```python
from build123d import *

# Parameters (mm, degrees)
BOSS_EXTRUDE1_DEPTH = 13.5
CUT_EXTRUDE1_DEPTH  = 19.454335534
SKETCH14_R          = 1.65
SKETCH14_R_2        = 1.483994527
BOSS_EXTRUDE3_DEPTH = 9.4
CUT_EXTRUDE7_DEPTH  = 43.344584395
FILLET2_R           = 2
CUT_EXTRUDE8_DEPTH  = 4
CUT_EXTRUDE9_DEPTH  = 5.4
CHAMFER2_SIZE       = 12
CHAMFER2_SIZE_2     = 6
CHAMFER3_SIZE       = 6
CHAMFER3_SIZE_2     = 12
SKETCH18_R          = 14.026707194
CUT_EXTRUDE10_DEPTH = 3
CUT_EXTRUDE11_DEPTH = 1


with BuildPart() as part:
    # Sketch1 → Boss-Extrude1 (new body)
    with BuildSketch(Plane.ZY):
        with BuildLine():
            Line((-9.5, 8.25), (-9.5, -8.25))
            Line((-9.5, -8.25), (0, -8.25))
            ThreePointArc((0, -8.25), (8.25, 0), (0, 8.25))
            Line((0, 8.25), (-9.5, 8.25))
        make_face()
    extrude(amount=BOSS_EXTRUDE1_DEPTH)

    # Sketch7 → Cut-Extrude1 (cut, through all)
    with BuildSketch(Plane.ZY.offset(13.5)):
        with BuildLine():
            Line((13.481907846, 13.481907846), (4.313351365, 4.313351365))
            ThreePointArc((4.313351365, 4.313351365), (-5.89214754, 1.578796175), (1.578796175, -5.89214754))
            Line((1.578796175, -5.89214754), (4.934720763, -18.416628609))
            Line((4.934720763, -18.416628609), (13.481907846, 13.481907846))
        make_face()
    extrude(amount=-CUT_EXTRUDE1_DEPTH, mode=Mode.SUBTRACT)

    # Sketch14 → Boss-Extrude3 (add)
    with BuildSketch(Plane(origin=(0, 0, -9.5), x_dir=(-1, 0, 0), z_dir=(0, 0, -1))):
        with BuildLine():
            Line((4.039848555, 24.201794753), (-19.358847021, 9.109670469))
            Line((-19.358847021, 9.109670469), (-19.131451731, 4.496469334))
            Line((-19.131451731, 4.496469334), (-15.022604709, 2.386798865))
            Line((-15.022604709, 2.386798865), (0, 12.07635684))
            Line((0, 12.07635684), (0, 8.25))
            Line((0, 8.25), (13.5, 8.25))
            Line((13.5, 8.25), (13.5, 12.07635684))
            Line((13.5, 12.07635684), (28.522604709, 2.386798865))
            Line((28.522604709, 2.386798865), (32.631451731, 4.496469334))
            Line((32.631451731, 4.496469334), (32.858847021, 9.109670469))
            Line((32.858847021, 9.109670469), (9.460151445, 24.201794753))
            ThreePointArc((9.460151445, 24.201794753), (6.75, 25), (4.039848555, 24.201794753))
        make_face()
        with Locations((6.75, 20)):
            Circle(SKETCH14_R, mode=Mode.SUBTRACT)
        with Locations((-15.25, 7)):
            Circle(SKETCH14_R_2, mode=Mode.SUBTRACT)
        with Locations(Location((28.75, 7, 0), (0, 0, 180))):
            Circle(SKETCH14_R_2, mode=Mode.SUBTRACT)
    extrude(amount=-BOSS_EXTRUDE3_DEPTH)

    # Sketch15 → Cut-Extrude7 (cut, through all)
    with BuildSketch(Plane.XY.offset(-0.1)):
        Polygon((0, 8.25), (-10.401710887, 8.25), (0, 10.084102275), align=None)
        Polygon((-13.5, 10.242254565), (-13.5, 12.07635684), (-3.098289113, 12.07635684), align=None)
    extrude(amount=-CUT_EXTRUDE7_DEPTH, mode=Mode.SUBTRACT)

    # Fillet2
    fillet2_edges = [part.edges().sort_by_distance(p)[0] for p in [
        (0, 10.084102275, -4.8),
        (-13.5, 10.242254565, -4.8),
    ]]
    fillet(fillet2_edges, radius=FILLET2_R)

    # Sketch16 → Cut-Extrude8 (cut)
    with BuildSketch(Plane(origin=(0, 0, -9.5), x_dir=(-1, 0, 0), z_dir=(0, 0, -1))):
        Polygon((6.75, 16.651368439), (9.65, 18.325684219), (9.65, 21.674315781), (6.75, 23.348631561), (3.85, 21.674315781), (3.85, 18.325684219), align=None)
    extrude(amount=-CUT_EXTRUDE8_DEPTH, mode=Mode.SUBTRACT)

    # Sketch17 → Cut-Extrude9 (cut)
    with BuildSketch(Plane.XY.offset(-0.1)):
        with BuildLine():
            Line((19.131451731, 4.496469334), (19.358847021, 9.109670469))
            Line((19.358847021, 9.109670469), (17.418121156, 10.361435802))
            ThreePointArc((17.418121156, 10.361435802), (11.888564198, 9.168121156), (13.081878844, 3.638564198))
            Line((13.081878844, 3.638564198), (15.022604709, 2.386798865))
            Line((15.022604709, 2.386798865), (19.131451731, 4.496469334))
        make_face()
        with BuildLine():
            Line((-32.631451731, 4.496469334), (-28.522604709, 2.386798865))
            Line((-28.522604709, 2.386798865), (-26.581878844, 3.638564198))
            ThreePointArc((-26.581878844, 3.638564198), (-25.388564198, 9.168121156), (-30.918121156, 10.361435802))
            Line((-30.918121156, 10.361435802), (-32.858847021, 9.109670469))
            Line((-32.858847021, 9.109670469), (-32.631451731, 4.496469334))
        make_face()
    extrude(amount=-CUT_EXTRUDE9_DEPTH, mode=Mode.SUBTRACT)

    # Chamfer2
    # the kernel refuses this chamfer: 12, 6 mm, written as the material it takes off along each edge
    with BuildSketch(Plane(origin=(-28.75, 7, -0.1), x_dir=(-0.8386519680093931, -0.5446676753342096, 0), z_dir=(-0.5446676753342096, 0.8386519680093931, 0))) as chamfer2_piece_1_section:
        Polygon((4 + CHAMFER2_SIZE, 0), (4, -CHAMFER2_SIZE_2), (4, 0), align=None)
    chamfer2_piece_1 = revolve(axis=Axis((-28.75, 7, -0.1), (0, 0, 1)), revolution_arc=359.64, mode=Mode.PRIVATE)
    chamfer2_piece_1 = split(chamfer2_piece_1, bisect_by=Plane(origin=(-24.520519127, 4.968138188, -1.544016366), z_dir=(-0.5420302889814643, 0.8403589505840171, 0)), keep=Keep.TOP, mode=Mode.PRIVATE)
    chamfer2_piece_1 = split(chamfer2_piece_1, bisect_by=Plane(origin=(-24.679235885, 5.214211241, -5.5), z_dir=(0, 0, 1)), keep=Keep.TOP, mode=Mode.PRIVATE)
    add(chamfer2_piece_1, mode=Mode.SUBTRACT)

    # Chamfer3
    # the kernel refuses this chamfer: 12, 6 mm, written as the material it takes off along each edge
    with BuildSketch(Plane(origin=(15.25, 7, -0.1), x_dir=(0.8420576391550663, -0.5393875530085916, 0), z_dir=(-0.5393875530085916, -0.8420576391550663, 0))) as chamfer3_piece_1_section:
        Polygon((4, -CHAMFER3_SIZE), (4 + CHAMFER3_SIZE_2, 0), (4, 0), align=None)
    chamfer3_piece_1 = revolve(axis=Axis((15.25, 7, -0.1), (0, 0, 1)), revolution_arc=359.64, mode=Mode.PRIVATE)
    chamfer3_piece_1 = split(chamfer3_piece_1, bisect_by=Plane(origin=(8.890128565, 11.795128101, -5.5), z_dir=(0, 0, 1)), keep=Keep.TOP, mode=Mode.PRIVATE)
    chamfer3_piece_1 = split(chamfer3_piece_1, bisect_by=Plane(origin=(0, 11.795128101, -1.99911645), z_dir=(1, 0, 0)), keep=Keep.TOP, mode=Mode.PRIVATE)
    add(chamfer3_piece_1, mode=Mode.SUBTRACT)

    # Sketch18 → Cut-Extrude10 (cut)
    with BuildSketch(Plane.XY.offset(-0.1)):
        with Locations((-6.75, 28.841468874)):
            Circle(SKETCH18_R)
    extrude(amount=-CUT_EXTRUDE10_DEPTH, mode=Mode.SUBTRACT)

    # Sketch19 → Cut-Extrude11 (cut)
    with BuildSketch(Plane.XY.offset(-5.5)):
        Polygon((-31.564052505, 5.184940267), (-28.585138414, 3.655429177), (-25.77108591, 5.47048891), (-25.935947495, 8.815059733), (-28.914861586, 10.344570823), (-31.72891409, 8.52951109), align=None)
        Polygon((18.064052505, 5.184940267), (18.22891409, 8.52951109), (15.414861586, 10.344570823), (12.435947495, 8.815059733), (12.27108591, 5.47048891), (15.085138414, 3.655429177), align=None)
    extrude(amount=-CUT_EXTRUDE11_DEPTH, mode=Mode.SUBTRACT)


solid = part.part
```
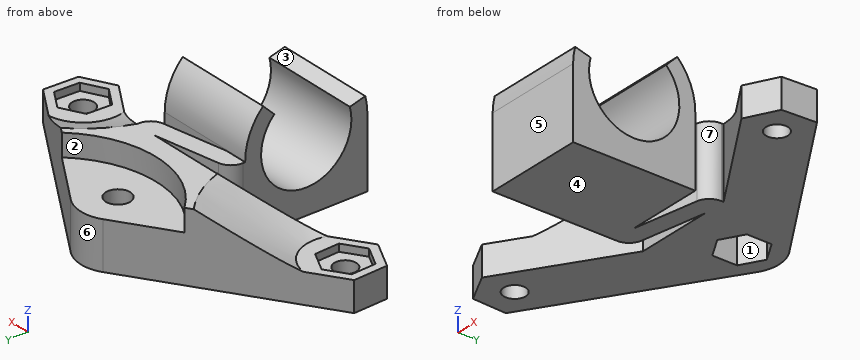
Check sheet for the modelled part. Datum: model origin and axes. Units: mm. Face numbers are marked on the shaded views. A direction names the side the tool comes from. Round coordinates to 2 decimals unless told otherwise and drop trailing zeros. Loops run counter-clockwise (first coordinate to the right, second up) from the corner with the lowest first, then second, coordinate; pieces in that order, holes last. Notation, with made-up numbers: (12, 24.5) -> (50, 24.5) arc R29 ccw to (50, 63.5) -> close; hole circle Ø11 at (-39, 72). An arc over 180 degrees is marked (long way). Write item = value, one per line. Start each with the question number.
1) Sectioned sample at B-B, the plane y = 20. Record the cut outline in (x, z).
2) Thickness scan on probe 1 along X at (y, z) = (8, -7); probe 2 along X at (y, z) = (-7, -1.5); probe 3 along Z at (x, y) = (-3, 0). Record the ranges inside material, lowest first.
3) Release check for a two-part mould opening along Y. For the marked faces 4, 5, 6 and 7 record: released by +Y, released by -Y, zero draft, split by the parting line, or undercut.
4) Gauge pin test, flat ends, axial feed: pin 1 Ø5 at (x, y) = (-7, 18) entering from +Z; pin 2 Ø1 at (x, y) = (-23, 10.5) entering from +Z; pin 3 Ø9 at (x, y) = (-10, 14) entering from +Z. Record the tip position at first contact, or that the pin passes through.
5) Set-up check for the marked faces 1, 2 and 3: record each of +Z, -Z, +X, -X, +Y, -Y from which the full face is reachable in a straight line by a thin tool's end or side.
6) Sectioned sample at D-D, the plane y = 0. Record the cut outline in (x, z).
7) Sectioned sample at C-C, the plane y = 7. State how many separate pieces and enclosed holes the cut face has, plus the area to 3 significant figures.
8) Sectioned sample at A-A, the plane z = -4. Record the cut outline in (x, y), plus the area to 3 significant figures.
Results are:
q1.outline = (-15.97, -9.5) -> (-9.65, -9.5) -> (-9.65, -5.5) -> (-8.4, -5.5) -> (-8.4, -3.1) -> (-15.97, -3.1) -> close; (-5.1, -5.5) -> (-3.85, -5.5) -> (-3.85, -9.5) -> (2.47, -9.5) -> (2.47, -3.1) -> (-5.1, -3.1) -> close
q2.probe_1 = -32.8 to -29.85, -27.65 to -19.82, -13.5 to 0, 6.32 to 14.15, 16.35 to 19.3
q2.probe_2 = -13.5 to 0
q2.probe_3 = -9.5 to -6.1
q3.face_4 = zero draft
q3.face_5 = released by -Y
q3.face_6 = released by +Y
q3.face_7 = undercut
q4.pin_1 = -3.1
q4.pin_2 = -4.48
q4.pin_3 = -0.1
q5.face_1 = -Z
q5.face_2 = +Z, +Y
q5.face_3 = +Z, +X, -X
q6.outline = (-13.5, -9.5) -> (0, -9.5) -> (0, -6.1) -> (-13.5, -6.1) -> close
q7.separate_pieces = 5
q7.enclosed_holes = 0
q7.area = 251 mm^2
q8.outline = (-24.9, 14.24) arc R8.2 cw to (-20.57, 7.52) -> (-13.5, 12.08) -> (-3.1, 12.08) -> (-11.85, 10.53) arc R2 ccw to (-13.5, 8.56) -> (-13.5, 4.61) -> (0, 4.61) -> (0, 8.25) -> (-10.4, 8.25) -> (-1.65, 9.79) arc R2 ccw to (0, 11.76) -> (0, 12.08) -> (7.07, 7.52) arc R8.2 cw to (11.4, 14.24) -> (-4.04, 24.2) arc R5 ccw to (-9.46, 24.2) -> close; (-13.5, -8.25) -> (0, -8.25) -> (0, -4.61) -> (-13.5, -4.61) -> close; hole circle Ø3.3 at (-6.75, 20)
q8.area = 442 mm^2
